Part model, mm, in its own coordinate system. A direction names the side the tool comes from. Give positions to 0.01 mm unless a question says otherwise; leave off trailing zeros. Loops run counter-clockwise (first coordinate to the right, second up) from the corner with the lowest first, then second, coordinate; pieces in that order, holes last. Notation, with made-up numbers: M 51.5,30.25 L 92.5,30.25 A13 ccw 92.5,40.25 Z; hole C -26,68.5 d3. An arc over 180 degrees is marked long. Answer in a Markdown table with one row per item.
from build123d import *

# Parameters (mm, degrees)
F1_DEPTH = 20
F2_R     = 19.99999
F3_R     = 10
F5_DEPTH = 10
F6_R     = 10
F7_DEPTH = 30
F9_D     = 10
F9_DEPTH = 10.001


# Not quite as in the source:
# - a fillet or chamfer is up to 0.001 mm smaller than in the source, because OpenCascade refuses the exact size


with BuildPart() as f1:
    # F0 (on Right) → F1 (new body, symmetric)
    with BuildSketch(Plane.YZ):
        Polygon((-60, 0), (0, 0), (0, 50), (-10, 50), (-10, 10), (-60, 10), align=None)
    extrude(amount=F1_DEPTH, both=True)

    # F2 (radius 20 in the source; OpenCascade refuses exactly that, so slightly less here)
    f2_edges = [f1.edges().sort_by_distance(p)[0] for p in [
        (-20, -60, 5),
        (20, -60, 5),
    ]]
    fillet(f2_edges, radius=F2_R)

    # F3
    f3_edges = [f1.edges().sort_by_distance(p)[0] for p in [
        (-20, -5, 50),
        (20, -5, 50),
    ]]
    fillet(f3_edges, radius=F3_R)

    # F4 (on face) → F5 (join)
    with BuildSketch(Plane.XY.offset(10)):
        with BuildLine():
            Line((-10, -10), (-10, -22.6794919243))
            ThreePointArc((-10, -22.6794919243), (-17.3205105757, -30.0000043301), (-20, -40.00001))
            ThreePointArc((-20, -40.00001), (-14.1421320882, -54.1421391593), (0, -60))
            ThreePointArc((0, -60), (14.1421320882, -54.1421391593), (20, -40.00001))
            ThreePointArc((20, -40.00001), (17.3205105757, -30.0000043301), (10, -22.6794919243))
            Line((10, -22.6794919243), (10, -10))
            Line((10, -10), (-10, -10))
        make_face()
    extrude(amount=F5_DEPTH)

    # F6 (on face) → F7 (join)
    with BuildSketch(Plane.XY.offset(20)):
        with Locations((0, -40)):
            Circle(F6_R)
    extrude(amount=F7_DEPTH)

    # F9 (through all, one way)
    with BuildSketch(Plane.XZ.offset(10)):
        with Locations((10, 40), (-10, 40)):
            Circle(F9_D / 2)
    extrude(amount=-F9_DEPTH, mode=Mode.SUBTRACT)


solid = f1.part
(1) Saw through at C-C (x = -7). Write the cut outline in (y, z) (3 decimals), plus the area to 3 significant figures.
Recorded:
| item | result |
|---|---|
| outline | M -58.735,0 L 0,0 L 0,36 L -10,36 L -10,20 L -32.859,20 L -32.859,50 L -47.141,50 L -47.141,20 L -58.735,20 Z; M -10,44 L 0,44 L 0,50 L -10,50 Z |
| area | 1,820 mm^2 |
(2) Which spindle directions (+Z, -Z, +X, -X, +Y, -Y) get a long thin tool onto all of the face, cutting with end or side? Do faces 5 (the face through (20, -11, 7)), 6 (the face through (10, -16, 15)), 7 (the face through (0, -29, 20)), 8 (the face through (-16, -18, 10)). Say none if no direction does.
Recorded:
| item | result |
|---|---|
| face 5 | +Z, -Z, +X, +Y, -Y |
| face 6 | +Z, +X |
| face 7 | +Z |
| face 8 | +Z, -X |
(3) Saw through at A-A (y = -7). Write the cut outline in (x, z), plus the area to 3 significant figures.
Recorded:
| item | result |
|---|---|
| outline | M -20,0 L 20,0 L 20,40 A10 ccw 10,50 L -10,50 A10 ccw -20,40 Z; hole C -10,40 d10; hole C 10,40 d10 |
| area | 1,800 mm^2 |
(4) Saw through at B-B (z = 30.5). Write the cut outline in (x, y).
Recorded:
| item | result |
|---|---|
| outline | M -20,-10 L 20,-10 L 20,0 L -20,0 Z; C 0,-40 d20 |
(5) Saw through at D-D (y = -33). Write the cut outline in (x, z) (3 decimals), plus the area to 3 significant figures.
Recorded:
| item | result |
|---|---|
| outline | M -20,0 L 20,0 L 20,10 L 18.735,10 L 18.735,20 L 7.141,20 L 7.141,50 L -7.141,50 L -7.141,20 L -18.735,20 L -18.735,10 L -20,10 Z |
| area | 1,200 mm^2 |
(6) Pin check, flat tips, straight feed: pin 1 Ø3 at (x, z) = (-6.5, 7.5) entering from -Y; pin 2 Ø5 at (y, z) = (-32.5, 15.5) entering from -X; pin 3 Ø3 at (x, y) = (-17, -22.5) entering from +Z. Stop position of each tip, or through.
Recorded:
| item | result |
|---|---|
| pin 1 | stops at y = -59.36 |
| pin 2 | stops at x = -19.36 |
| pin 3 | stops at z = 10 |
(7) Drill centre lines: line 1 along X through (y, z) = (-7, 36); line 2 along X through (y, z) = (-6, 36.5); line 3 along Z through (x, y) = (-10, -7). Where is each one in solid material? Low to high.
Recorded:
| item | result |
|---|---|
| line 1 | x = -20 to -13, -7 to 7, 13 to 20 |
| line 2 | x = -20 to -13.57, -6.43 to 6.43, 13.57 to 20 |
| line 3 | z = 0 to 35, 45 to 50 |
(8) Pull direction X, two halves, no side cores. Call faces 1 (the face through (-7, -5, 44)), 2 (the face through (17.15, -5.07, 46.99)), 3 (the face through (13, -5, 44)), 4 (the face through (16, -18, 10)): +X half, -X half, draft (parallel to the pull), parting line (faces both ways), or undercut.
Recorded:
| item | result |
|---|---|
| face 1 | undercut |
| face 2 | +X half |
| face 3 | undercut |
| face 4 | draft |
